Input: part model. Units: mm. Frame: model coordinates. Face numbers are marked on the shaded views. Give positions to 0.01 mm unless a question says otherwise; leave off trailing zeros. Loops run counter-clockwise (first coordinate to the right, second up) from the corner with the lowest first, then second, coordinate; pieces in that order, holes last. Notation, with made-up numbers: (12, 29) -> (51, 29) arc R20 cw to (51, 59) -> close; hole circle Ø10 at (53, 51). An arc over 180 degrees is marked (long way). One line per question, with ' | ' between items.
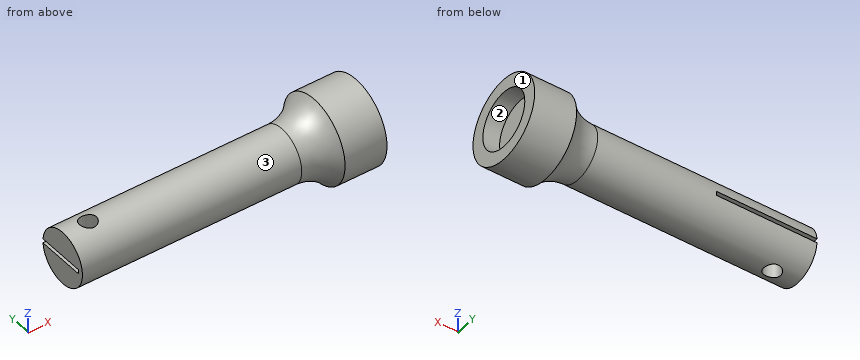
from build123d import *

# Parameters (mm, degrees)
SKETCH_1_R               = 3.2
EXTRUDE_1_DEPTH          = 30
SKETCH_2_W               = 0.5
SKETCH_2_H               = 6.454336116
CUT_EXTRUDE_1_DEPTH      = 12
CUT_EXTRUDE_2_DEPTH      = 10
CUT_EXTRUDE_2_DEPTH_BACK = 10
SKETCH_3_R               = 1
SKETCH_6_R               = 5
EXTRUDE_2_DEPTH          = 5
FILLET_1_R               = 5
SKETCH_7_R               = 3.4
CUT_EXTRUDE_3_DEPTH      = 2


with BuildPart() as part:
    # 草图1 → 凸台-拉伸1 (new body)
    with BuildSketch(Plane(origin=(0, 0, 0), x_dir=(0, 0, -1), z_dir=(1, 0, 0))):
        Circle(SKETCH_1_R)
    extrude(amount=EXTRUDE_1_DEPTH)

    # 草图2 → 切除-拉伸1 (cut)
    with BuildSketch(Plane.ZY):
        with Locations((0, 0.634798729)):
            Rectangle(SKETCH_2_W, SKETCH_2_H)
    extrude(amount=-CUT_EXTRUDE_1_DEPTH, mode=Mode.SUBTRACT)

    # 草图3 → 切除-拉伸2 (cut, two sides: drawn at the far end of the back side and taken through both)
    with BuildSketch(Plane(origin=(0, 0, 0.25), x_dir=(-1, 0, 0), z_dir=(0, 0, -1)).offset(-CUT_EXTRUDE_2_DEPTH_BACK)):
        with Locations(Location((-3, -0.004890286, 0), (0, 0, 180))):
            Circle(SKETCH_3_R)
    extrude(amount=CUT_EXTRUDE_2_DEPTH + CUT_EXTRUDE_2_DEPTH_BACK, mode=Mode.SUBTRACT)

    # 草图6 → 凸台-拉伸2 (add)
    with BuildSketch(Plane(origin=(30, 0, 0), x_dir=(0, 0, -1), z_dir=(1, 0, 0))):
        Circle(SKETCH_6_R)
    extrude(amount=EXTRUDE_2_DEPTH)

    # 圆角1
    # the kernel refuses this fillet: 5 mm, written as the material it adds along each edge
    with BuildSketch(Plane(origin=(30, 0, 0), x_dir=(0, 0, -1), z_dir=(0, -1, 0))) as fillet_1_piece_1:
        with BuildLine():
            CenterArc((8.2, -3.841874542), FILLET_1_R, 129.7918195, 50.2081805)
            Line((3.2, -3.841874542), (3.1, -3.841874542))
            Line((3.1, -3.841874542), (3.1, 0))
            Line((3.1, 0), (3.2, 0.1))
            ThreePointArc((3.2, 0.1), (4.1, 0.1), (4.936, 0.076837491))
            Line((4.936, 0.076837491), (5, 0))
        make_face()
    revolve(axis=Axis((30, 0, 0), (1, 0, 0)))

    # 草图7 → 切除-拉伸3 (cut)
    with BuildSketch(Plane(origin=(35, 0, 0), x_dir=(0, 0, -1), z_dir=(1, 0, 0))):
        Circle(SKETCH_7_R)
    extrude(amount=-CUT_EXTRUDE_3_DEPTH, mode=Mode.SUBTRACT)


solid = part.part
1. Ray query, line 1 along X through (y, z) = (-0.5, -2.5); line 2 along Y through (x, z) = (33.6, 0); line 3 along X through (y, z) = (-0.25, -0.75). Return the intervals inside material, ascending. Write a range as from..to.
Determined:
line 1: x = 0..2.13, 3.87..33 | line 2: y = -5..-3.4, 3.4..5 | line 3: x = 0..2.03, 3.97..33
2. Pull-direction query (Z, two-part tool) for the marked faces 1, 2 and 3; classes: pulls with the +Z half, pulls with the -Z half, needs draft (parallel to the pull), parting line crosses it, or undercut.
Determined:
face 1: needs draft | face 2: undercut | face 3: parting line crosses it
3. Section query B-B (x = 21.5). Output: boundary loops of the cut face in (y, z), then the cut area to 3 significant figures.
Determined:
outline: circle Ø6.4 at (0, 0) | area: 32.2 mm2
4. Pin query (flat end, axial travel): P1, Ø1.8, axis at x = 3, y = 0, coming from the +Z side; P2, Ø4.5, axis at x = 8.5, y = 0.5, coming from the +Z side; P3, Ø4.5, axis at x = 5.5, y = 1.5, coming from the -Z side; P4, Ø4, axis at x = 7, y = 3.5, coming from the +Z side. Return the tip coordinate at first contact, or that it passes through.
Determined:
P1: passes through | P2: stops at z = 3.2 | P3: stops at z = -3.2 | P4: stops at z = 2.83
5. Section query C-C (x = 11.5). Output: boundary loops of the cut face in (y, z).
Determined:
outline: (-2.59, -0.25) -> (-2.59, 0.25) -> (3.19, 0.25) arc R3.2 ccw (long way) to (3.19, -0.25) -> close
6. Section query A-A (x = 3). Output: boundary loops of the cut face in (y, z).
Determined:
outline: (-2.59, -0.25) -> (-2.59, 0.25) -> (-1, 0.25) -> (-1, 3.04) arc R3.2 ccw to (-1, -3.04) -> (-1, -0.25) -> close; (1, -3.04) arc R3.2 ccw to (3.19, -0.25) -> (1, -0.25) -> close; (1, 0.25) -> (3.19, 0.25) arc R3.2 ccw to (1, 3.04) -> close
